```python
from build123d import *

# Parameters (mm, degrees)
SKETCH3_RX          = 2.216625444
SKETCH3_RY          = 1.445625289
CUT_EXTRUDE1_DEPTH  = 5
FILLET1_R           = 2
BOSS_EXTRUDE1_DEPTH = 1.5


with BuildPart() as part:
    # Sketch1 → Revolve1 (revolve)
    with BuildSketch(Plane(origin=(0, 0, 0), x_dir=(1, 0, 0), z_dir=(0, 1, 0)), mode=Mode.PRIVATE) as revolve1_sk:
        Polygon((5.5, 0), (-5.5, 0), (-5.5, 15.5), (3.5, 15.5), (3.5, 18), (5.5, 18), (6, 18), (6, 17.5), (5.5, 17.5), (5, 16.5), (5, 16), (7, 12), (7, 6), (6, 3.845161331), (6, 3.018549032), (7, 2.554477167), (7, 0), align=None)
    revolve(revolve1_sk.sketch.rotate(Axis((-25, 0, 0), (1, 0, 0)), 180), axis=Axis((-25, 0, 0), (1, 0, 0)))

    # Sketch3 → Cut-Extrude1 (cut, symmetric)
    with BuildSketch(Plane(origin=(7, 0, 0), x_dir=(0, 0, -1), z_dir=(1, 0, 0))):
        with Locations(Location((0, 13.926190288), (0, 0, 0))):
            Ellipse(SKETCH3_RX, SKETCH3_RY)
        with Locations(Location((13.244594021, 4.303429466), (0, 0, 108))):
            Ellipse(SKETCH3_RX, SKETCH3_RY)
        with Locations(Location((8.185609272, -11.26652461), (0, 0, 36))):
            Ellipse(SKETCH3_RX, SKETCH3_RY)
        with Locations(Location((-8.185609272, -11.26652461), (0, 0, -36))):
            Ellipse(SKETCH3_RX, SKETCH3_RY)
        with Locations(Location((-13.244594021, 4.303429466), (0, 0, 72))):
            Ellipse(SKETCH3_RX, SKETCH3_RY)
    extrude(amount=CUT_EXTRUDE1_DEPTH, both=True, mode=Mode.SUBTRACT)

    # Fillet1
    # the kernel refuses this fillet: 2 mm, written as the material it takes off along each edge
    with BuildSketch(Plane(origin=(7, 0, 0), x_dir=(0, 0, 1), z_dir=(0, 1, 0))) as fillet1_piece_1:
        with BuildLine():
            CenterArc((1.286498225, -2), FILLET1_R, 30, 60)
            Line((1.286498225, 0), (1.286498225, 0.04))
            Line((1.286498225, 0.04), (2.554477167, 0.04))
            Line((2.554477167, 0.04), (2.590760489, 0.016838069))
            ThreePointArc((2.590760489, 0.016838069), (2.822796422, -0.483161931), (3.053190048, -0.98))
            Line((3.053190048, -0.98), (3.018549032, -1))
        make_face()
    revolve(axis=Axis((7, 0, 0), (1, 0, 0)), mode=Mode.SUBTRACT)

    # Sketch4 → Boss-Extrude1 (add)
    with BuildSketch(Plane(origin=(7, 0, 0), x_dir=(0, 0, -1), z_dir=(1, 0, 0))):
        Polygon((7.749630704, 3.250124219), (8.80400944, 3.865505525), (8.798262965, 5.086314949), (7.738137753, 5.691743068), (6.683759016, 5.076361762), (6.689505491, 3.855552338), align=None)
        Polygon((1.060125212, 8.336439169), (1.054378737, 9.557248593), (-0.005746475, 10.162676712), (-1.060125212, 9.547295406), (-1.054378737, 8.326485982), (0.005746475, 7.721057863), align=None)
        Polygon((6.689505491, -5.086314949), (7.749630704, -5.691743068), (8.80400944, -5.076361762), (8.798262965, -3.855552338), (7.738137753, -3.250124219), (6.683759016, -3.865505525), align=None)
        Polygon((-1.060125212, -8.336439169), (-1.054378737, -9.557248593), (0.005746475, -10.162676712), (1.060125212, -9.547295406), (1.054378737, -8.326485982), (-0.005746475, -7.721057863), align=None)
        Polygon((-7.749630704, -3.250124219), (-8.80400944, -3.865505525), (-8.798262965, -5.086314949), (-7.738137753, -5.691743068), (-6.683759016, -5.076361762), (-6.689505491, -3.855552338), align=None)
        Polygon((-6.689505491, 5.086314949), (-7.749630704, 5.691743068), (-8.80400944, 5.076361762), (-8.798262965, 3.855552338), (-7.738137753, 3.250124219), (-6.683759016, 3.865505525), align=None)
    extrude(amount=BOSS_EXTRUDE1_DEPTH)


solid = part.part
```
Part model, mm, in its own coordinate system. A direction names the side the tool comes from. Give positions to 0.01 mm unless a question says otherwise; leave off trailing zeros. Write each loop counter-clockwise with the first axis right and the second up, starting at its lowest first coordinate (ties: lowest second). Pieces come first, ordered by that corner, then holes. Notation, with made-up numbers: (-11, 37) -> (46, 37) arc R26 ccw to (46, 66) -> close; hole circle Ø1 at (83, -11). An arc over 180 degrees is marked (long way). Put each result on its own line as item: value. Start each with the question number.
Item 1: Cut at A-A (x = -1.5). List the corners of the cut face in (y, z), then the cut area to 3 significant figures.
Item 2: Pull direction Z, two halves, no side cores. Call faces 1 (the face through (7.74, -5.39, 7.22)), 2 (the face through (7.74, -5.38, 8.28)), 3 (the face through (7.74, 9.856, -0.532)): pulls with the +Z half, pulls with the -Z half, needs draft (parallel to the pull), parting line crosses it, or undercut.
Item 3: Wall check: L1, parallel to Y at x = 5.75, z = -1; L2, parallel to Y at x = 5.95, z = 0; L3, parallel to X at y = -4, z = -4.5. Give the ranges that are in metal, low to high. Write a range as [from, to].
Item 4: Which spindle directions (+Z, -Z, +X, -X, +Y, -Y) get a long thin tool onto all of the face, cutting with end or side? Do faces 4 (the face through (7, 0, 0)), 5 (the face through (3.5, -15, -5)), 6 (the face through (7.74, 9.859, 0.526)), 7 (the face through (7.74, 5.39, -7.22)). Say none if no direction does.
Item 5: Cut at B-B (x = 4.5). State how many separate pieces and enclosed holes the cut face has, then the cut area to 3 significant figures.
Item 6: Pin check, flat tips, straight feed: pin 1 Ø0.9 at (y, z) = (3.5, 13) entering from +X; pin 2 Ø8.5 at (y, z) = (-1.5, -1) entering from +X; pin 3 Ø1 at (x, y) = (1.5, 3.5) entering from +Z; pin 4 Ø6 at (y, z) = (-7, -5.5) entering from +X. Stop position of each tip, or through.
Answer list:
1. outline: circle Ø31 at (0, 0)
1. area: 755 mm2
2. face 1: undercut
2. face 2: pulls with the +Z half
2. face 3: pulls with the -Z half
3. L1: y = [-17.97, -17.47], [-14.47, 12.64], [17.47, 17.97]
3. L2: y = [-18, -17.5], [-14.1, 12.48], [17.5, 18]
3. L3: x = [-5.5, 7]
4. face 4: +Z, -Z, +X
4. face 5: -X
4. face 6: +Z, +X, +Y
4. face 7: +X, +Y
5. separate pieces: 1
5. enclosed holes: 5
5. area: 968 mm2
6. pin 1: stops at x = 2
6. pin 2: stops at x = 7
6. pin 3: stops at z = 15.21
6. pin 4: stops at x = 8.5
